Here's how the part is built. I have some questions about the finished solid (model axes, mm). Face numbers are marked on the shaded views. A direction names the side the tool comes from. Coordinates: 2 decimals unless noted, no trailing zeros. Write each loop counter-clockwise with the first axis right and the second up, starting at its lowest first coordinate (ties: lowest second). Pieces come first, ordered by that corner, then holes.
Item 1: If we section it at B-B (z = 1.5): Please give me the cut outline in (x, y), then the cut area to 3 significant figures.
Item 2: If we section it at D-D (z = 6.75): Please give me the cut outline in (x, y).
Item 3: If I drill on line 1 (Y direction, x = 0, z = 11.3); line 2 (Z direction, x = 4.5, y = 49.5); line 3 (X direction, y = 9.5, z = 10), over which ranges is the centre line in solid material (lowest first)?
Item 4: We'd pull the mould along Z, two halves only. Please class the marked faces 1, 2 and 3: +Z half, -Z half, draft (parallel to the pull), parting line (faces both ways), or undercut.
Item 5: If we section it at C-C (y = 22): Please give me the cut outline in (x, z).
Item 6: I'm going to push flat-ended pins straight in: pin 1 Ø1.8 at (x, z) = (-1.5, 5.5) entering from +Y; pin 2 Ø4 at (y, z) = (-22, 3.5) entering from -X; pin 3 Ø4 at (y, z) = (40.5, 4) entering from +X. Where does each tip first touch, or does it pass through?
Item 7: For the marked faces 4, 5, 6 and 7, which set-ups out of +Z, -Z, +X, -X, +Y, -Y let a thin tool reach every point of the face, with its end or its side?
Item 8: If we section it at A-A (x = 0): Please give me the cut outline in (y, z), then the cut area to 3 significant figures.
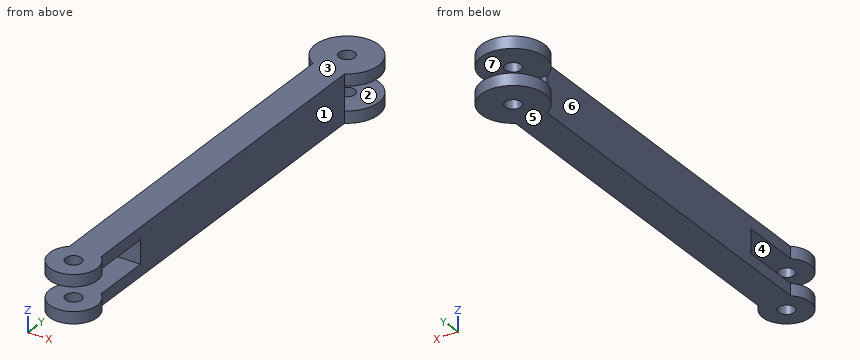
from build123d import *

# Parameters (mm, degrees)
SALIENTE_EXTRUIR1_DEPTH = 12
CROQUIS3_R              = 2
CORTAR_EXTRUIR1_DEPTH   = 63.903673209
CROQUIS4_W              = 30
CROQUIS4_H              = 6
CORTAR_EXTRUIR2_DEPTH   = 14
CROQUIS5_W              = 8
CROQUIS5_H              = 6
CORTAR_EXTRUIR3_DEPTH   = 15
CROQUIS8_W              = 30
CROQUIS8_H              = 6
CORTAR_EXTRUIR6_DEPTH   = 39


with BuildPart() as part:
    # Croquis1 → Saliente-Extruir1 (new body)
    with BuildSketch(Plane.XY):
        with BuildLine():
            Line((-4, 46.299830407), (-4, -46.299830407))
            ThreePointArc((-4, -46.299830407), (0, -56.771966362), (4, -46.299830407))
            Line((4, -46.299830407), (4, 46.299830407))
            ThreePointArc((4, 46.299830407), (0, 61.228033638), (-4, 46.299830407))
        make_face()
    extrude(amount=SALIENTE_EXTRUIR1_DEPTH)

    # Croquis3 → Cortar-Extruir1 (cut, through all)
    with BuildSketch(Plane.XY.offset(12)):
        with Locations((0, 53.228033638)):
            Circle(CROQUIS3_R)
        with Locations((0, -50.771966362)):
            Circle(CROQUIS3_R)
    extrude(amount=-CORTAR_EXTRUIR1_DEPTH, mode=Mode.SUBTRACT)

    # Croquis4 → Cortar-Extruir2 (cut)
    with BuildSketch(Plane(origin=(0, -46.299830407, 0), x_dir=(1, 0, 0), z_dir=(0, 1, 0))):
        with Locations((0, -6)):
            Rectangle(CROQUIS4_W, CROQUIS4_H)
    extrude(amount=-CORTAR_EXTRUIR2_DEPTH, mode=Mode.SUBTRACT)

    # Croquis5 → Cortar-Extruir3 (cut)
    with BuildSketch(Plane.XZ.offset(46.299830407)):
        with Locations((0, 6)):
            Rectangle(CROQUIS5_W, CROQUIS5_H)
    extrude(amount=-CORTAR_EXTRUIR3_DEPTH, mode=Mode.SUBTRACT)

    # Croquis8 → Cortar-Extruir6 (cut)
    with BuildSketch(Plane(origin=(0, 46.299830407, 0), x_dir=(1, 0, 0), z_dir=(0, 1, 0))):
        with Locations((0, -6)):
            Rectangle(CROQUIS8_W, CROQUIS8_H)
    extrude(amount=CORTAR_EXTRUIR6_DEPTH, mode=Mode.SUBTRACT)


solid = part.part
Answer list:
1. outline: (-4, -46.3) arc R6 ccw (long way) to (4, -46.3) - (4, 46.3) arc R8 ccw (long way) to (-4, 46.3) - close; hole circle Ø4 at (0, -50.77); hole circle Ø4 at (0, 53.23)
1. area: 1,020 mm2
2. outline: (-4, -31.3) - (4, -31.3) - (4, 46.3) - (-4, 46.3) - close
3. line 1: y = -56.77 to -52.77, -48.77 to 51.23, 55.23 to 61.23
3. line 2: z = 0 to 3, 9 to 12
3. line 3: x = -4 to 4
4. face 1: draft
4. face 2: undercut
4. face 3: +Z half
5. outline: (-4, 0) - (4, 0) - (4, 12) - (-4, 12) - close
6. pin 1: stops at y = 46.3
6. pin 2: stops at x = -4
6. pin 3: stops at x = 4
7. face 4: +X, -X, -Y
7. face 5: -Z, +X, -X, +Y, -Y
7. face 6: +Z, -Z, -X
7. face 7: +X, -X, +Y
8. outline: (-56.77, 0) - (-52.77, 0) - (-52.77, 3) - (-56.77, 3) - close; (-56.77, 9) - (-52.77, 9) - (-52.77, 12) - (-56.77, 12) - close; (-48.77, 0) - (51.23, 0) - (51.23, 3) - (46.3, 3) - (46.3, 9) - (51.23, 9) - (51.23, 12) - (-48.77, 12) - (-48.77, 9) - (-31.3, 9) - (-31.3, 3) - (-48.77, 3) - close; (55.23, 0) - (61.23, 0) - (61.23, 3) - (55.23, 3) - close; (55.23, 9) - (61.23, 9) - (61.23, 12) - (55.23, 12) - close
8. area: 1,130 mm2
